Check sheet for the modelled part. Datum: model origin and axes. Units: mm. A direction names the side the tool comes from. Round coordinates to 2 decimals unless told otherwise and drop trailing zeros. Write each loop counter-clockwise with the first axis right and the second up, starting at its lowest first coordinate (ties: lowest second). Pieces come first, ordered by that corner, then holes. Notation, with made-up numbers: (61.5, 55.25) - (65.5, 55.25) arc R12 cw to (65.5, 67.25) - close; hole circle Ø9 at (-24, -13). An arc over 180 degrees is marked (long way). Answer as a JSON object with one key per item and string values. Group by question number.
Item 1: Gauge pin test, flat ends, axial feed: P1, Ø3.5, axis at x = -14.16, y = 9.16, coming from the +Z side; P2, Ø1, axis at x = 31.5, z = 1.5, coming from the -Y side; P3, Ø0.6, axis at y = -39, z = 0.5, coming from the +X side; P4, Ø1, axis at x = 31, z = 0.5, coming from the +Y side. Record the tip position at first contact, or that the pin passes through.
Item 2: Set-up check for faces 5 (the flat face through (30.224, 31, 1)), 6 (the flat face through (5.324, 28.877, 0.986)), 7 (the flat face through (30.059, -32, 1)): record each of +Z, -Z, +X, -X, +Y, -Y from which the full face is reachable in a straight line by a thin tool's end or side.
Item 3: Thickness scan on line 1 (X direction, y = -34, z = 0.7); line 2 (Y direction, x = 12, z = 0.95); line 3 (Y direction, x = 21, z = 1.8). Record the ranges inside material, lowest first.
Item 4: Sectioned sample at D-D on y = 22.5. Record the boundary of the cut face in (x, z), plus the area to 3 significant figures.
Item 5: Sectioned sample at A-A on z = 0.55. Record the boundary of the cut face in (x, y), plus the area to 3 significant figures.
Item 6: Sectioned sample at C-C on x = -28.5. Record the boundary of the cut face in (y, z), plus the area to 3 significant figures.
Item 7: Release check for a two-part mould opening along Y. For faces 1 (the flat face through (20, -37.82, 1)), 2 (the cylindrical face through (-17.19, -26.72, 0.99)), 3 (the cylindrical face through (21.37, 0.36, 0.99)), 4 (the flat face through (18.112, 32.416, 0.986)) record: pulls with the +Y half, pulls with the -Y half, needs draft (parallel to the pull), parting line crosses it, or undercut.
Item 8: Sectioned sample at B-B on y = -1.5. Record the boundary of the cut face in (x, z).
```python
from build123d import *

# Parameters (mm, degrees)
EXTRUDE_1_DEPTH          = 2
SKETCH_3_R               = 2.25
CUT_EXTRUDE_1_DEPTH      = 2
CUT_EXTRUDE_1_DEPTH_BACK = 10


with BuildPart() as part:
    # 草图2 → 凸台-拉伸1 (new body)
    with BuildSketch(Plane.XY):
        Polygon((30.22420133, 24.680203113), (30.22420133, 36.760203113), (5.656415061, 27.949194211), (4.981241965, 29.831783197), (-42.083482687, 12.952455799), (-41.408309591, 11.069866813), (-64.940671917, 2.630203113), (-64.940671917, -37.369796887), (-39.940671917, -37.369796887), (-39.940671917, -39.819796887), (10.059328083, -39.819796887), (10.059328083, -37.819796887), (30.059328083, -37.819796887), (30.059328083, -25.319796887), (32.22420133, -25.319796887), (32.22420133, 24.680203113), align=None)
    extrude(amount=EXTRUDE_1_DEPTH)

    # 草图3 → 切除-拉伸1 (cut, two sides)
    with BuildSketch(Plane.XY) as cut_extrude_1_sk:
        with Locations((-14.162495237, 9.155291089)):
            Circle(SKETCH_3_R)
        with Locations((19.22420133, -0.319796887)):
            Circle(SKETCH_3_R)
        with Locations((-14.940671917, -26.819796887)):
            Circle(SKETCH_3_R)
    extrude(amount=CUT_EXTRUDE_1_DEPTH, mode=Mode.SUBTRACT)
    extrude(cut_extrude_1_sk.sketch, amount=-CUT_EXTRUDE_1_DEPTH_BACK, mode=Mode.SUBTRACT)


solid = part.part
```
Completed:
{
 "1": {"P1": "through", "P2": "y = -25.32", "P3": "x = 10.06", "P4": "y = 24.68"},
 "2": {"face 5": "+Z, -Z, +X, +Y", "face 6": "+Z, -Z, +Y", "face 7": "+Z, -Z, +X, -Y"},
 "3": {"line 1": "-64.94 to 30.06", "line 2": "-37.82 to 30.22", "line 3": "-37.82 to -1.7, 1.06 to 33.45"},
 "4": {"outline": "(-15.46, 0) - (32.22, 0) - (32.22, 2) - (-15.46, 2) - close", "area": "95.4 mm²"},
 "5": {"outline": "(-64.94, -37.37) - (-39.94, -37.37) - (-39.94, -39.82) - (10.06, -39.82) - (10.06, -37.82) - (30.06, -37.82) - (30.06, -25.32) - (32.22, -25.32) - (32.22, 24.68) - (30.22, 24.68) - (30.22, 36.76) - (5.66, 27.95) - (4.98, 29.83) - (-42.08, 12.95) - (-41.41, 11.07) - (-64.94, 2.63) - close; hole circle Ø4.5 at (-14.94, -26.82); hole circle Ø4.5 at (-14.16, 9.16); hole circle Ø4.5 at (19.22, -0.32)", "area": "5,710 mm²"},
 "6": {"outline": "(-39.82, 0) - (17.82, 0) - (17.82, 2) - (-39.82, 2) - close", "area": "115 mm²"},
 "7": {"face 1": "pulls with the -Y half", "face 2": "undercut", "face 3": "undercut", "face 4": "pulls with the +Y half"},
 "8": {"outline": "(-64.94, 0) - (17.31, 0) - (17.31, 2) - (-64.94, 2) - close; (21.14, 0) - (32.22, 0) - (32.22, 2) - (21.14, 2) - close"}
}
